Geometry: final body of the model. Coordinates: model frame, mm. A direction names the side the tool comes from. Give positions to 0.01 mm unless a question says otherwise; leave off trailing zeros. Loops run counter-clockwise (first coordinate to the right, second up) from the corner with the lowest first, then second, coordinate; pieces in that order, holes last.
from build123d import *

# Parameters (mm, degrees)
PAD_DEPTH    = 20
SKETCH001_R  = 6
PAD001_DEPTH = 1.5
SKETCH002_R  = 3
PAD002_DEPTH = 7
SKETCH003_R  = 2
POCKET_DEPTH = 32.201
SKETCH004_W  = 4
SKETCH004_H  = 7
PAD003_DEPTH = 8


with BuildPart() as part:
    # Sketch → Pad (new body)
    with BuildSketch(Plane.XY):
        Polygon((0, 0), (40.6, 0), (40.6, 28), (47.5, 28), (47.5, 32.2), (40.6, 32.2), (40.6, 41), (0, 41), (0, 32.2), (-6.9, 32.2), (-6.9, 28), (0, 28), align=None)
    extrude(amount=PAD_DEPTH)

    # Sketch001 (on Face8 of Pad) → Pad001 (join)
    with BuildSketch(Plane(origin=(0, 41, 0), x_dir=(-1, 0, 0), z_dir=(0, 1, 0))):
        with Locations((-9, 10)):
            Circle(SKETCH001_R)
    extrude(amount=PAD001_DEPTH)

    # Sketch002 (on Face16 of Pad001) → Pad002 (join)
    with BuildSketch(Plane(origin=(0, 42.5, 0), x_dir=(-1, 0, 0), z_dir=(0, 1, 0))):
        with Locations((-9, 10)):
            Circle(SKETCH002_R)
    extrude(amount=PAD002_DEPTH)

    # Sketch003 (on Face10 of Pad002) → Pocket (cut, through all)
    with BuildSketch(Plane(origin=(0, 32.2, 0), x_dir=(-1, 0, 0), z_dir=(0, 1, 0))):
        with Locations((4.2, 15)):
            Circle(SKETCH003_R)
        with Locations((4.2, 5)):
            Circle(SKETCH003_R)
        with Locations((-44.8, 5)):
            Circle(SKETCH003_R)
        with Locations((-44.8, 15)):
            Circle(SKETCH003_R)
    extrude(amount=-POCKET_DEPTH, mode=Mode.SUBTRACT)

    # Sketch004 (on Face9 of Pocket) → Pad003 (join)
    with BuildSketch(Plane.YZ.offset(40.6)):
        with Locations((5, 10)):
            Rectangle(SKETCH004_W, SKETCH004_H)
    extrude(amount=PAD003_DEPTH)


solid = part.part
Item 1: Section query D-D on z = 15. Return loops of the section in (x, y).
Values follow:
outline: (-6.9, 28) - (-6.2, 28) - (-6.2, 32.2) - (-6.9, 32.2) - close; (-2.2, 28) - (0, 28) - (0, 0) - (40.6, 0) - (40.6, 28) - (42.8, 28) - (42.8, 32.2) - (40.6, 32.2) - (40.6, 41) - (12.32, 41) - (12.32, 42.5) - (5.68, 42.5) - (5.68, 41) - (0, 41) - (0, 32.2) - (-2.2, 32.2) - close; (46.8, 28) - (47.5, 28) - (47.5, 32.2) - (46.8, 32.2) - close
Item 2: Ray query, probe 1 along Z at (x, y) = (44.8, 31.1); probe 2 along X at (y, z) = (30, 6.75); probe 3 along Y at (x, z) = (44.5, 10.5). Return the intervals inside material, ascending.
Values follow:
probe 1: z = 0 to 3, 7 to 13, 17 to 20
probe 2: x = -6.9 to -5.17, -3.23 to 43.83, 45.77 to 47.5
probe 3: y = 3 to 7, 28 to 32.2
Item 3: Set-up query: faces 4 (the face through (40.6, 37, 10)), 5 (the face through (0, 14, 10)), 6 (the face through (-3, 32.2, 10)), 7 (the face through (45, 5, 6.5)), 8 (the face through (45, 3, 10)). Return all of +Z, -Z, +X, -X, +Y, -Y with unobstructed straight access to the full face (end or side cutting, diameter ignored); none if empty.
Values follow:
face 4: +Z, -Z, +X, +Y
face 5: +Z, -Z, -X, -Y
face 6: +Z, -Z, -X, +Y
face 7: -Z, +X, -Y
face 8: +Z, -Z, +X, -Y
Item 4: Pin query (flat end, axial travel): pin 1 (5.5 mm diameter, centred on x = -2, z = 6.5, fed in from -Y); pin 2 (4.5 mm diameter, centred on x = -4.2, z = 5, fed in from -Y); pin 3 (1 mm diameter, centred on y = 14.5, z = 9.5, fed in from -X); pin 4 (10 mm diameter, centred on y = 20.5, z = 13.5, fed in from +X). Return the tip coordinate at first contact, or that it passes through.
Values follow:
pin 1: stops at y = 0
pin 2: stops at y = 28
pin 3: stops at x = 0
pin 4: stops at x = 40.6
Item 5: Draft query along Z for faces 1 (the face through (20, 0, 10)), 2 (the face through (45, 5, 13.5)), 3 (the face through (46.798, 30.129, 5.088)). Return one class per face: +Z half, -Z half, draft (parallel to the pull), parting line (faces both ways), or undercut.
Values follow:
face 1: draft
face 2: +Z half
face 3: undercut
Item 6: Section query B-B on y = 31. Return loops of the section in (x, z).
Values follow:
outline: (-6.9, 0) - (47.5, 0) - (47.5, 20) - (-6.9, 20) - close; hole circle Ø4 at (-4.2, 5); hole circle Ø4 at (-4.2, 15); hole circle Ø4 at (44.8, 5); hole circle Ø4 at (44.8, 15)
Item 7: Section query A-A on x = -4.2. Return loops of the section in (y, z), plus the area to 3 significant figures.
Values follow:
outline: (28, 0) - (32.2, 0) - (32.2, 3) - (28, 3) - close; (28, 7) - (32.2, 7) - (32.2, 13) - (28, 13) - close; (28, 17) - (32.2, 17) - (32.2, 20) - (28, 20) - close
area: 50.4 mm2
Item 8: Section query C-C on x = 9. Return loops of the section in (y, z), plus the area to 3 significant figures.
Values follow:
outline: (0, 0) - (41, 0) - (41, 4) - (42.5, 4) - (42.5, 7) - (49.5, 7) - (49.5, 13) - (42.5, 13) - (42.5, 16) - (41, 16) - (41, 20) - (0, 20) - close
area: 880 mm2
